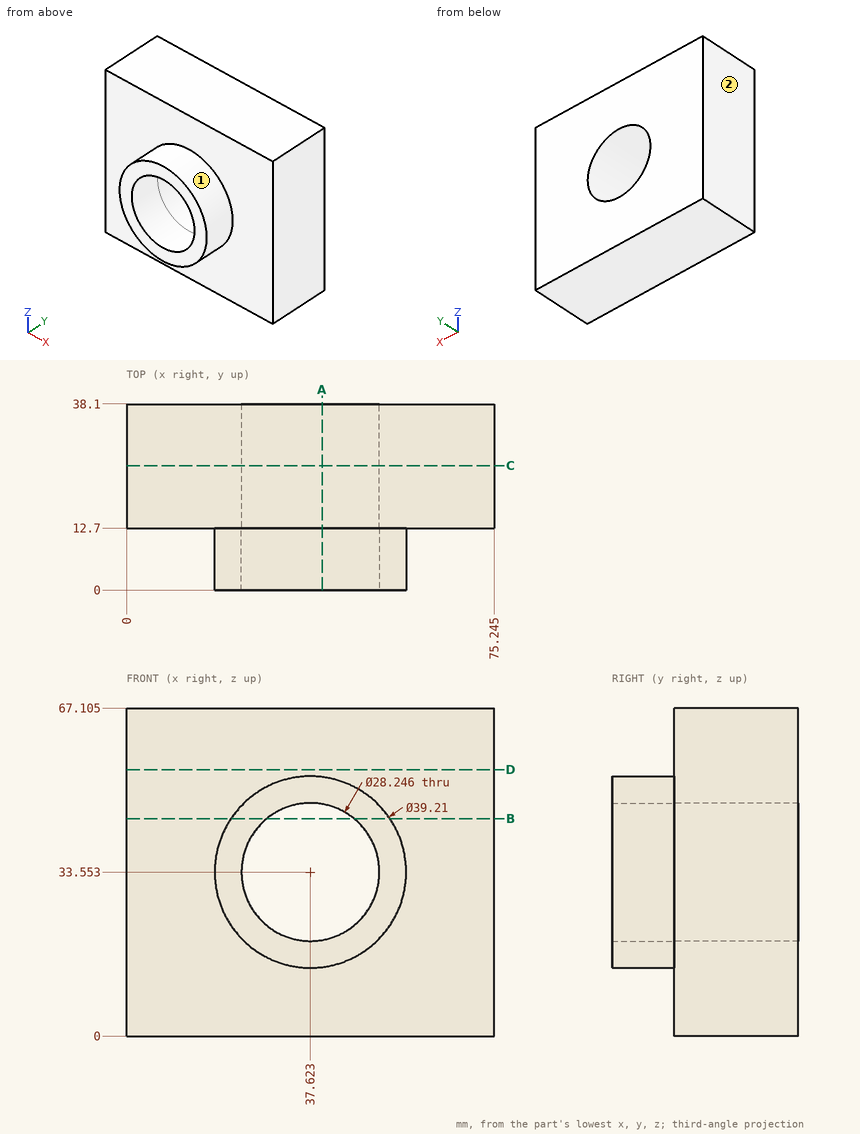
Job drawing, mm, ordinate dimensions from the low corner. One solid piece. A direction names the side the tool comes from. Round coordinates to 2 decimals unless told otherwise and drop trailing zeros. Loops run counter-clockwise (first coordinate to the right, second up) from the corner with the lowest first, then second, coordinate; pieces in that order, holes last. Notation, with made-up numbers: M 5,80 L 58,80 A10 ccw 58,91 Z; hole C 74,47 d1. An arc over 180 degrees is marked long. One line per question, with ' | ' between items. Start each with the question number.
Item 1: Wall check: line 1 (Y direction, x = 43.5, z = 62); line 2 (Z direction, x = 36, y = 10.5) (1 decimal); line 3 (Z direction, x = 46.5, y = 21) (1 decimal). Give the ranges that are in metal, low to high.
Item 2: Cut at A-A, the plane x = 40. Write the cut outline in (y, z) (1 decimal), plus the area to 3 significant figures.
Item 3: Cut at C-C, the plane y = 25.5. Write the cut outline in (x, z) (1 decimal).
Item 4: Cut at D-D, the plane z = 54.5. Write the cut outline in (x, y) (1 decimal).
Item 5: Pin check, flat tip, straight feed: pin 1 Ø22.5 at (x, z) = (37.62, 33.55) entering from -Y. Stop position of the tip, or through.
Item 6: Which spindle directions (+Z, -Z, +X, -X, +Y, -Y) get a long thin tool onto all of the face, cutting with end or side? Do the marked faces 1 and 2. Say none if no direction does.
Item 7: Cut at B-B, the plane z = 44.5. Write the cut outline in (x, y) (1 decimal), plus the area to 3 significant figures.
Responses:
1) line 1: y = 12.7 to 38.1 | line 2: z = 14 to 19.5, 47.6 to 53.1 | line 3: z = 0 to 22.6, 44.5 to 67.1
2) outline: M 0,14.1 L 12.7,14.1 L 12.7,0 L 38.1,0 L 38.1,19.6 L 0,19.6 Z; M 0,47.5 L 38.1,47.5 L 38.1,67.1 L 12.7,67.1 L 12.7,53 L 0,53 Z | area: 1,140 mm²
3) outline: M 0,0 L 75.2,0 L 75.2,67.1 L 0,67.1 Z; hole C 37.6,33.6 d28.2
4) outline: M 0,12.7 L 75.2,12.7 L 75.2,38.1 L 0,38.1 Z
5) pin 1: passes through
6) face 1: -Y | face 2: +Z, -Z, -X, +Y, -Y
7) outline: M 0,12.7 L 21.4,12.7 L 21.4,0 L 28.7,0 L 28.7,38.1 L 0,38.1 Z; M 46.5,0 L 53.9,0 L 53.9,12.7 L 75.2,12.7 L 75.2,38.1 L 46.5,38.1 Z | area: 1,640 mm²
